from build123d import *

# Parameters (mm, degrees)
SKETCH_1_W      = 40
SKETCH_1_H      = 80
EXTRUDE_1_DEPTH = 3.5
FILLET_1_R      = 4.5
FILLET_2_R      = 3


with BuildPart() as part:
    # 草图1 → 凸台-拉伸1 (new body)
    with BuildSketch(Plane.XY):
        with Locations((68.192883988, 40)):
            Rectangle(SKETCH_1_W, SKETCH_1_H)
    extrude(amount=EXTRUDE_1_DEPTH)

    # 圆角1
    fillet_1_edges = [part.edges().sort_by_distance(p)[0] for p in [
        (48.192883988, 0, 1.75),
        (48.192883988, 80, 1.75),
        (88.192883988, 80, 1.75),
        (88.192883988, 0, 1.75),
    ]]
    fillet(fillet_1_edges, radius=FILLET_1_R)

    # 圆角2
    fillet_2_edges = [part.edges().sort_by_distance(p)[0] for p in [
        (68.192883988, 0, 3.5),
        (48.192883988, 40, 3.5),
        (88.192883988, 40, 3.5),
        (68.192883988, 80, 3.5),
        (86.874864503, 78.681980515, 3.5),
        (49.510903472, 78.681980515, 3.5),
        (86.874864503, 1.318019485, 3.5),
        (49.510903472, 1.318019485, 3.5),
    ]]
    fillet(fillet_2_edges, radius=FILLET_2_R)


solid = part.part
Part model, mm, in its own coordinate system. Round coordinates to 2 decimals unless told otherwise and drop trailing zeros. Write each loop counter-clockwise with the first axis right and the second up, starting at its lowest first coordinate (ties: lowest second). Pieces come first, ordered by that corner, then holes. Notation, with made-up numbers: (13.25, 10.25) - (31.25, 10.25) arc R24 ccw to (31.25, 20.25) - close; hole circle Ø7 at (36, 73.25). An arc over 180 degrees is marked (long way). Use CSV: the item, a comma, the result in double quotes.
Item 1: Wall check: L1, parallel to Y at x = 75.5, z = 0.65; L2, parallel to Z at x = 51, y = 69; L3, parallel to Y at x = 66, z = 2.05. Give the ranges that are in metal, low to high.
Results list:
L1,"y = 0 to 80"
L2,"z = 0 to 3.49"
L3,"y = 0.43 to 79.57"
Item 2: Flat gauge pin, fed straight in: P1, Ø1.5, axis at y = 68, z = 2.5, coming from the +X side. Where does the tip first touch, or does it go through?
Results list:
P1,"stops at x = 87.92"
Item 3: Pull direction Z, two halves, no side cores. Call faces 1 (the flat face through (68, 41, 0)), 2 (the cylindrical face through (49.48, 1.35, 0.25)), 3 (the cylindrical face through (67.98, 79.1, 2.64)): pulls with the +Z half, pulls with the -Z half, needs draft (parallel to the pull), parting line crosses it, or undercut.
Results list:
face 1,"pulls with the -Z half"
face 2,"needs draft"
face 3,"pulls with the +Z half"
Item 4: Slice it at A-A, the plane y = 6.5. Write the cut outline in (x, z).
Results list:
outline,"(48.19, 0) - (88.19, 0) - (88.19, 0.5) arc R3 ccw to (85.19, 3.5) - (51.19, 3.5) arc R3 ccw to (48.19, 0.5) - close"
